```python
from build123d import *

# Parameters (mm, degrees)
F0_W           = 88.9
F0_H           = 12.7
F1_DEPTH       = 50.8
F2_W           = 19.05
F2_H           = 15.875
F3_DEPTH       = 6.35
F5_START       = 12.7
F4_R           = 6.35
F5_DEPTH       = 63.5
F6_W           = 38.1
F6_H           = 44.45
F7_DEPTH       = 50.8
F9_D           = 6.35
F9_CSINK_D     = 12.7
F9_CSINK_ANGLE = 90


with BuildPart() as f1:
    # F0 (on Front) → F1 (new body)
    with BuildSketch(Plane.XZ):
        with Locations((44.45, 6.35)):
            Rectangle(F0_W, F0_H)
    extrude(amount=F1_DEPTH)

    # F2 (on Top) → F3 (join)
    with BuildSketch(Plane.XY):
        with Locations((79.375, 7.9375)):
            Rectangle(F2_W, F2_H)
        with Locations((79.375, -58.7375)):
            Rectangle(F2_W, F2_H)
        with Locations((9.525, -58.7375)):
            Rectangle(F2_W, F2_H)
        with Locations((9.525, 7.9375)):
            Rectangle(F2_W, F2_H)
        with BuildLine():
            ThreePointArc((19.05, 15.875), (9.525, 25.4), (0, 15.875))
            Line((0, 15.875), (19.05, 15.875))
        make_face()
        with BuildLine():
            Line((19.05, -66.675), (0, -66.675))
            ThreePointArc((0, -66.675), (9.525, -76.2), (19.05, -66.675))
        make_face()
        with BuildLine():
            ThreePointArc((88.9, 15.875), (79.375, 25.4), (69.85, 15.875))
            Line((69.85, 15.875), (88.9, 15.875))
        make_face()
        with BuildLine():
            Line((88.9, -66.675), (69.85, -66.675))
            ThreePointArc((69.85, -66.675), (79.375, -76.2), (88.9, -66.675))
        make_face()
    extrude(amount=F3_DEPTH)

    # F4 (on Right) → F5 (join)
    with BuildSketch(Plane.YZ.offset(F5_START)):
        Polygon((-50.8, 0), (0, 0), (0, 12.5690720878), (-12.7, 12.5690720878), (-38.1, 12.5690720878), (-50.8, 12.5690720878), align=None)
        with BuildLine():
            Line((-38.1, 12.5690720878), (-12.7, 12.5690720878))
            Line((-12.7, 12.5690720878), (-12.7, 40.0571599603))
            ThreePointArc((-12.7, 40.0571599603), (-25.4, 52.7571599603), (-38.1, 40.0571599603))
            Line((-38.1, 40.0571599603), (-38.1, 12.5690720878))
        make_face()
        with Locations((-25.4, 40.0571599603)):
            Circle(F4_R, mode=Mode.SUBTRACT)
    extrude(amount=F5_DEPTH)

    # F6 (on Front) → F7 (cut)
    with BuildSketch(Plane.XZ):
        with Locations((44.45, 34.925)):
            Rectangle(F6_W, F6_H)
    extrude(amount=F7_DEPTH, mode=Mode.SUBTRACT)

    # F9 (through all)
    with Locations(Plane.XY.offset(6.35)):
        with Locations((9.525, -66.675), (79.375, -66.675), (9.525, 15.875), (79.375, 15.875)):
            CounterSinkHole(F9_D / 2, F9_CSINK_D / 2, counter_sink_angle=F9_CSINK_ANGLE)


solid = f1.part
```
Read the model definition and answer for the solid it produces. Units are mm, in the model's axes. A direction names the side the tool comes from. Give positions to 0.01 mm unless a question says otherwise; leave off trailing zeros. Order: outer loops, then holes, each group sorted by start corner. A loop starts at its lowest first (then second) coordinate and runs counter-clockwise, first axis right, second up. Notation, with made-up numbers: (27, 48.25) -> (57, 48.25) arc R35 cw to (57, 82.25) -> close; hole circle Ø1 at (-12.5, 41.25). An arc over 180 degrees is marked (long way). One line per item, written item: value. Start each with the question number.
(1) Flat-ended cylindrical pins translate along their axes: P1, Ø1.5, axis at x = 47, y = -17.5, coming from the +Z side; P2, Ø15, axis at x = 77, y = 18.5, coming from the +Z side; P3, Ø6.5, axis at x = 19.5, z = 24.5, coming from the +Y side. Find the tip coordinate at first contact, or state that the pin passes through.
(2) The part is cut by section B-B (y = -25.4). Determine the outline of the cut face in (x, z).
(3) The part is cut by section D-D (x = 35). Determine the outline of the cut face in (y, z), and give its area (3 significant figures).
(4) A tool of negligible diameter and unlimited length cuts with its end or side. For faces 4 (the flat face through (79, 7, 6.35)), 5 (the flat face through (44, 0, 8)), 6 (the flat face through (25.4, -25, 28)), 7 (the flat face through (77, -60, 6.35)), 8 (the flat face through (19.05, -59, 3)), from which of +Z, -Z, +X, -X, +Y, -Y can it reach the whole face along a straight path? Write none if from no direction.
(5) For a pull along Y with two mould halves and no side action, classify faces 1 (the cylindrical face through (18.961, -25.121, 52.754)), 2 (the flat face through (76.2, -26, 29)), 3 (the cylindrical face through (76.347, 16.829, 1.565)) as released by +Y, released by -Y, zero draft, split by the parting line, or undercut.
(6) Straight lines are drawn through the part: L1, parallel to Z at x = 66.5, y = -25.4; L2, parallel to X at y = -24, z = 31; L3, parallel to Y at x = 69, z = 15. For each, find the intervals that lie inside material, in ascending order.
(7) The part is cut by section A-A (z = 18). Determine the outline of the cut face in (x, y), and give its area (3 significant figures).
(8) The part is cut by section C-C (z = 42). Determine the outline of the cut face in (x, y).
Taken from the geometry:
1. P1: z = 12.7
1. P2: z = 6.35
1. P3: y = -12.7
2. outline: (0, 0) -> (88.9, 0) -> (88.9, 12.7) -> (76.2, 12.7) -> (76.2, 33.71) -> (63.5, 33.71) -> (63.5, 12.7) -> (25.4, 12.7) -> (25.4, 33.71) -> (12.7, 33.71) -> (12.7, 12.7) -> (0, 12.7) -> close; (12.7, 46.41) -> (25.4, 46.41) -> (25.4, 52.76) -> (12.7, 52.76) -> close; (63.5, 46.41) -> (76.2, 46.41) -> (76.2, 52.76) -> (63.5, 52.76) -> close
3. outline: (-50.8, 0) -> (0, 0) -> (0, 12.7) -> (-50.8, 12.7) -> close
3. area: 645 mm^2
4. face 4: +Z, +X, -X, +Y
4. face 5: +Z, +Y
4. face 6: +Z, +Y, -Y
4. face 7: +Z, +X, -X, -Y
4. face 8: +Z, -Z, -Y
5. face 1: split by the parting line
5. face 2: zero draft
5. face 3: undercut
6. L1: 0 to 33.71, 46.41 to 52.76
6. L2: 12.7 to 25.4, 63.5 to 76.2
6. L3: -38.1 to -12.7
7. outline: (12.7, -38.1) -> (25.4, -38.1) -> (25.4, -12.7) -> (12.7, -12.7) -> close; (63.5, -38.1) -> (76.2, -38.1) -> (76.2, -12.7) -> (63.5, -12.7) -> close
7. area: 645 mm^2
8. outline: (12.7, -37.95) -> (25.4, -37.95) -> (25.4, -31.45) -> (12.7, -31.45) -> close; (12.7, -19.35) -> (25.4, -19.35) -> (25.4, -12.85) -> (12.7, -12.85) -> close; (63.5, -37.95) -> (76.2, -37.95) -> (76.2, -31.45) -> (63.5, -31.45) -> close; (63.5, -19.35) -> (76.2, -19.35) -> (76.2, -12.85) -> (63.5, -12.85) -> close
